Autodesk Inventor part; units mm, degrees
ref_plane "YZ Plane" through (0, 0, 0) normal (1, 0, 0) x (0, 1, 0)
ref_plane "XZ Plane" through (0, 0, 0) normal (0, 1, 0) x (-1, 0, 0)
ref_plane "XY Plane" through (0, 0, 0) normal (0, 0, 1) x (1, 0, 0)
sketch "Skizze1" plane through (0, 0, 0) normal (1, 0, 0) x (0, 1, 0)
  line L0 (-60, 50) -> (60, 50)
  line L1 (60, 50) -> (60, -50)
  line L2 (60, -50) -> (-60, -50)
  line L3 (-60, -50) -> (-60, 50)
  line L4 (0, 37.4988) -> (0, -37.4988) construction
  line L5 (-78.3748, 0) -> (89.6252, 0) construction
  line L6 (-57.15, 46.36) -> (57.15, 46.36) construction
  line L7 (57.15, 46.36) -> (57.15, -46.36) construction
  line L8 (57.15, -46.36) -> (-57.15, -46.36) construction
  line L9 (-57.15, -46.36) -> (-57.15, 46.36) construction
  circle A0 centre (-57.15, 46.36) radius 1.25
  circle A1 centre (57.15, 46.36) radius 1.25
  circle A2 centre (-57.15, -46.36) radius 1.25
  circle A3 centre (57.15, -46.36) radius 1.25
  line L10 (-60, 50) -> (60.1722, 49.7926) construction
  line L11 (60.1722, 49.7926) -> (60, -50) construction
  line L12 (60, -50) -> (-60.1722, -49.7926) construction
  line L13 (-60.1722, -49.7926) -> (-60, 50) construction
  point P0 (0, 0)
  point P1 (0, 0)
  point P2 (0, 0)
  dimension "d0" = 120
  dimension "d1" = 100
  dimension "d4" = 2.5
  dimension "d5" = 114.3
  dimension "d6" = 92.72
extrude "Extrusion1" add sketch "Skizze1" along normal blind 2
properties part number "MotorController"
Read the model definition and answer for the solid it produces. Units are mm, in the model's axes. Coordinates: 2 decimals unless noted, no trailing zeros. Order: outer loops, then holes, each group sorted by start corner. A loop starts at its lowest first (then second) coordinate and runs counter-clockwise, first axis right, second up. Notation, with made-up numbers: M 41.25,-24 L 92.25,-24 A33 cw 92.25,15 Z; hole C 89,-35 d7. An arc over 180 degrees is marked long. Put each result on its own line as item: value. Start each with the question number.
Item 1: Section B-B, the plane y = -57.15 is taken. Determine the outline of the cut face in (x, z), plus the area to 3 significant figures.
Item 2: Consider probe 1 along Z at (x, y) = (0.45, 57.15). Determine where the line is inside the solid, lowest interval first. Write a range as [from, to].
Item 3: Section A-A, the plane z = -46.36 is taken. Determine the outline of the cut face in (x, y), plus the area to 3 significant figures.
Item 4: The mould has two halves that part along Z. Classify faces 1 (the face through (1, -57.3, -47.6)), 2 (the face through (0, -1, 1)): +Z half, -Z half, draft (parallel to the pull), parting line (faces both ways), or undercut.
Computed:
1. outline: M 0,-50 L 2,-50 L 2,-47.61 L 0,-47.61 Z; M 0,-45.11 L 2,-45.11 L 2,45.11 L 0,45.11 Z; M 0,47.61 L 2,47.61 L 2,50 L 0,50 Z
1. area: 190 mm2
2. probe 1: z = [-50, -47.61], [-45.11, 45.11], [47.61, 50]
3. outline: M 0,-60 L 2,-60 L 2,-58.4 L 0,-58.4 Z; M 0,-55.9 L 2,-55.9 L 2,55.9 L 0,55.9 Z; M 0,58.4 L 2,58.4 L 2,60 L 0,60 Z
3. area: 230 mm2
4. face 1: undercut
4. face 2: draft
